Verification items for the finished model (mm, model axes). A direction names the side the tool comes from. Coordinates: 2 decimals unless noted, no trailing zeros. Write each loop counter-clockwise with the first axis right and the second up, starting at its lowest first coordinate (ties: lowest second). Pieces come first, ordered by that corner, then holes. Notation, with made-up numbers: (82, -33) -> (136, -33) arc R31 cw to (136, 0) -> close; hole circle Ø9 at (67, -8). An arc over 180 degrees is marked (long way). Answer in a Markdown table with one row per item.
```python
from build123d import *

# Parameters (mm, degrees)
SKETCH1_R           = 2.4780875
BOSS_EXTRUDE1_DEPTH = 1.5875


with BuildPart() as part:
    # Sketch1 → Boss-Extrude1 (new body, symmetric)
    with BuildSketch(Plane(origin=(0, 0, 0), x_dir=(1, 0, 0), z_dir=(0, 1, 0))):
        Polygon((-15.9766, 12.8016), (15.9766, 12.8016), (15.9766, 4.8895), (19.1516, 4.8895), (19.1516, -4.8895), (15.9766, -4.8895), (15.9766, -12.8016), (-15.9766, -12.8016), (-15.9766, -4.8895), (-19.1516, -4.8895), (-19.1516, 4.8895), (-15.9766, 4.8895), align=None)
        Circle(SKETCH1_R, mode=Mode.SUBTRACT)
    extrude(amount=BOSS_EXTRUDE1_DEPTH, both=True)


solid = part.part
```
1. Sectioned sample at D-D, the plane z = -6.75. Record the cut outline in (x, y).
Findings below:
| item | result |
|---|---|
| outline | (-15.98, -1.59) -> (15.98, -1.59) -> (15.98, 1.59) -> (-15.98, 1.59) -> close |
2. Material ranges on probe 1 along X at (y, z) = (0.05, 0); probe 2 along Z at (x, y) = (0, -0.3); probe 3 along X at (y, z) = (-0.5, -8.25), recorded low to high. Write a range as from..to.
Findings below:
| item | result |
|---|---|
| probe 1 | x = -19.15..-2.48, 2.48..19.15 |
| probe 2 | z = -12.8..-2.48, 2.48..12.8 |
| probe 3 | x = -15.98..15.98 |
3. Release check for a two-part mould opening along X. For faces 1 (the face through (15.977, 0, 9)), 2 (the face through (-1.83, -0.02, -1.67)), 3 (the face through (-18, 0, 4.89)) record: released by +X, released by -X, zero draft, split by the parting line, or undercut.
Findings below:
| item | result |
|---|---|
| face 1 | released by +X |
| face 2 | undercut |
| face 3 | zero draft |
4. Go/stop test with flat-tipped pins: pin 1 (1.6 mm diameter, centred on y = -0.5, z = 7, fed in from +X); pin 2 (1.6 mm diameter, centred on x = 18, y = -0.5, fed in from -Z); pin 3 (1 mm diameter, centred on y = -0.5, z = 7, fed in from -X). Record where each tip stops, or that it passes through.
Findings below:
| item | result |
|---|---|
| pin 1 | stops at x = 15.98 |
| pin 2 | stops at z = -4.89 |
| pin 3 | stops at x = -15.98 |
5. Sectioned sample at B-B, the plane z = 0. Record the cut outline in (x, y), and give its area (3 significant figures).
Findings below:
| item | result |
|---|---|
| outline | (-19.15, -1.59) -> (-2.48, -1.59) -> (-2.48, 1.59) -> (-19.15, 1.59) -> close; (2.48, -1.59) -> (19.15, -1.59) -> (19.15, 1.59) -> (2.48, 1.59) -> close |
| area | 106 mm² |
6. Access from +Z, -Z, +X, -X, +Y, -Y to the whole of each face (thin tool, end or side, straight path). Record for faces 4 (the face through (-15.977, 0, -9)), 5 (the face through (-15.977, 0, 9)), 6 (the face through (18, 0, -4.89)).
Findings below:
| item | result |
|---|---|
| face 4 | -Z, -X, +Y, -Y |
| face 5 | +Z, -X, +Y, -Y |
| face 6 | -Z, +X, +Y, -Y |
7. Sectioned sample at A-A, the plane x = 0. Record the cut outline in (y, z), and give its area (3 significant figures).
Findings below:
| item | result |
|---|---|
| outline | (-1.59, -12.8) -> (1.59, -12.8) -> (1.59, -2.48) -> (-1.59, -2.48) -> close; (-1.59, 2.48) -> (1.59, 2.48) -> (1.59, 12.8) -> (-1.59, 12.8) -> close |
| area | 65.6 mm² |
8. Sectioned sample at C-C, the plane y = -1.15. Record the cut outline in (x, z).
Findings below:
| item | result |
|---|---|
| outline | (-19.15, -4.89) -> (-15.98, -4.89) -> (-15.98, -12.8) -> (15.98, -12.8) -> (15.98, -4.89) -> (19.15, -4.89) -> (19.15, 4.89) -> (15.98, 4.89) -> (15.98, 12.8) -> (-15.98, 12.8) -> (-15.98, 4.89) -> (-19.15, 4.89) -> close; hole circle Ø4.96 at (0, 0) |
